from build123d import *

# Parameters (mm, degrees)
SKETCH_R     = 12
PAD_DEPTH    = 5
SKETCH001_R  = 6
PAD001_DEPTH = 30
FILLET_R     = 4


with BuildPart() as part:
    # Sketch → Pad (new body)
    with BuildSketch(Plane.XY):
        with BuildLine():
            Line((-69, -75), (69, -75))
            ThreePointArc((69, -75), (73.242641, -73.242641), (75, -69))
            Line((75, -69), (75, 69))
            ThreePointArc((75, 69), (73.242641, 73.242641), (69, 75))
            Line((69, 75), (-69, 75))
            ThreePointArc((-69, 75), (-73.242641, 73.242641), (-75, 69))
            Line((-75, 69), (-75, -69))
            ThreePointArc((-75, -69), (-73.242641, -73.242641), (-69, -75))
        make_face()
        with Locations((-54, 54)):
            Circle(SKETCH_R, mode=Mode.SUBTRACT)
        with Locations((-18, 54)):
            Circle(SKETCH_R, mode=Mode.SUBTRACT)
        with Locations((18, 54)):
            Circle(SKETCH_R, mode=Mode.SUBTRACT)
        with Locations((54, 54)):
            Circle(SKETCH_R, mode=Mode.SUBTRACT)
        with Locations((-54, 18)):
            Circle(SKETCH_R, mode=Mode.SUBTRACT)
        with Locations((-18, 18)):
            Circle(SKETCH_R, mode=Mode.SUBTRACT)
        with Locations((18, 18)):
            Circle(SKETCH_R, mode=Mode.SUBTRACT)
        with Locations((54, 18)):
            Circle(SKETCH_R, mode=Mode.SUBTRACT)
        with Locations((-54, -18)):
            Circle(SKETCH_R, mode=Mode.SUBTRACT)
        with Locations((-18, -18)):
            Circle(SKETCH_R, mode=Mode.SUBTRACT)
        with Locations((18, -18)):
            Circle(SKETCH_R, mode=Mode.SUBTRACT)
        with Locations((54, -18)):
            Circle(SKETCH_R, mode=Mode.SUBTRACT)
        with Locations((-54, -54)):
            Circle(SKETCH_R, mode=Mode.SUBTRACT)
        with Locations((-18, -54)):
            Circle(SKETCH_R, mode=Mode.SUBTRACT)
        with Locations((18, -54)):
            Circle(SKETCH_R, mode=Mode.SUBTRACT)
        with Locations((54, -54)):
            Circle(SKETCH_R, mode=Mode.SUBTRACT)
    extrude(amount=PAD_DEPTH)

    # Sketch001 (on Face26 of Pad) → Pad001 (join)
    with BuildSketch(Plane.XY.offset(5)):
        with Locations((-69, 69)):
            Circle(SKETCH001_R)
        with Locations((69, 69)):
            Circle(SKETCH001_R)
        with Locations((69, -69)):
            Circle(SKETCH001_R)
        with Locations((-69, -69)):
            Circle(SKETCH001_R)
    extrude(amount=PAD001_DEPTH)

    # Fillet
    fillet_edges = [part.edges().sort_by_distance(p)[0] for p in [
        (0, -75, 0),
        (-75, 0, 0),
        (0, 75, 0),
        (75, 0, 0),
    ]]
    fillet(fillet_edges, radius=FILLET_R)


solid = part.part
CAD build for the part. Positions are in the model's coordinates, mm. Coordinates: 2 decimals unless noted, no trailing zeros. Write each loop counter-clockwise with the first axis right and the second up, starting at its lowest first coordinate (ties: lowest second). Pieces come first, ordered by that corner, then holes. Notation, with made-up numbers: M 20.25,70 L 72.25,70 A18 ccw 72.25,82 Z; hole C 4.25,-1.75 d10. An arc over 180 degrees is marked long. Return JSON: item names as keys, results as strings.
Item 1: Probe line 1 (Y direction, x = -17, z = 4); line 2 (Y direction, x = -54, z = 1); line 3 (X direction, y = -27, z = 3.5). List the from-to ranges inside material, lowest first. Write a range as from..to.
Findings below:
{"line 1": "y = -75..-65.96, -42.04..-29.96, -6.04..6.04, 29.96..42.04, 65.96..75", "line 2": "y = -73.65..-66, -42..-30, -6..6, 30..42, 66..73.65", "line 3": "x = -74.97..-61.94, -46.06..-25.94, -10.06..10.06, 25.94..46.06, 61.94..74.97"}
Item 2: Slice it at A-A, the plane x = 18. Write the cut outline in (y, z), and give its area (3 significant figures).
Findings below:
{"outline": "M -75,4 A4 ccw -71,0 L -66,0 L -66,5 L -75,5 Z; M -42,0 L -30,0 L -30,5 L -42,5 Z; M -6,0 L 6,0 L 6,5 L -6,5 Z; M 30,0 L 42,0 L 42,5 L 30,5 Z; M 66,0 L 71,0 A4 ccw 75,4 L 75,5 L 66,5 Z", "area": "263 mm2"}
Item 3: Drop a flat-ended pin along its axis: pin 1 Ø1 at (x, y) = (-33.5, 54) entering from +Z. Give the stop position or say it passes through.
Findings below:
{"pin 1": "stops at z = 5"}
Item 4: Two-plate mould, pull along X, no slides. Class faces 1 (the cylindrical face through (73.859, 0.966, 1.203)), 2 (the flat face through (-1, 1, 5)), 3 (the cylindrical face through (-0.966, 73.859, 1.203)): +X half, -X half, draft (parallel to the pull), parting line (faces both ways), or undercut.
Findings below:
{"face 1": "+X half", "face 2": "undercut", "face 3": "draft"}
Item 5: Slice it at C-C, the plane z = 21. Write the cut outline in (x, y).
Findings below:
{"outline": "C -69,-69 d12; C -69,69 d12; C 69,-69 d12; C 69,69 d12"}
